Work out the finished part from the listing and answer in its coordinate system (mm). Coordinates: 2 decimals unless noted, no trailing zeros. Loops run counter-clockwise (first coordinate to the right, second up) from the corner with the lowest first, then second, coordinate; pieces in that order, holes last. Notation, with made-up numbers: (18.5, 61) -> (75.5, 61) arc R30 ccw to (75.5, 92) -> close; hole circle Ø8 at (28.5, -27.5). An arc over 180 degrees is marked (long way). Use a Markdown table: item, result. Add a question column.
```python
from build123d import *

# Parameters (mm, degrees)
F0_W         = 90
F0_H         = 60
F1_DEPTH     = 3
F2_R         = 2.5
F3_DEPTH     = 2
F4_R         = 1.5
F5_DEPTH     = 5
F6_R         = 7
F7_DEPTH     = 2.5
F8_R         = 5.25
F8_R_2       = 2.1
F9_DEPTH     = 4.3
F10_DEPTH    = 5.5
F11_W        = 31.5768257218
F11_H        = 6.5
F12_DEPTH    = 3
F13_T1_DEPTH = 3
F14_SIZE     = 1.5
F15_R        = 5
F16_R        = 3


# Not quite as in the source:
# - a fillet or chamfer that OpenCascade refuses, or shapes differently, is made with other operations: its cross-section is extruded or revolved along the edge and cut away or added


with BuildPart() as f1:
    # F0 (on Top) → F1 (new body)
    with BuildSketch(Plane.XY):
        Rectangle(F0_W, F0_H)
    extrude(amount=F1_DEPTH)

    # F2 (on face) → F3 (join)
    with BuildSketch(Plane.XY.offset(3)):
        with Locations((-39, 24.5)):
            Circle(F2_R)
        with Locations((19, 24.5)):
            Circle(F2_R)
        with Locations((19, -24.5)):
            Circle(F2_R)
        with Locations((-39, -24.5)):
            Circle(F2_R)
    extrude(amount=F3_DEPTH)

    # F4 (on face) → F5 (cut, through all)
    with BuildSketch(Plane(origin=(0, 0, 0), x_dir=(1, 0, 0), z_dir=(0, 0, -1))):
        with Locations((-39, 24.5)):
            Circle(F4_R)
        with Locations((19, 24.5)):
            Circle(F4_R)
        with Locations((19, -24.5)):
            Circle(F4_R)
        with Locations((-39, -24.5)):
            Circle(F4_R)
    extrude(amount=-F5_DEPTH, mode=Mode.SUBTRACT)

    # F6 (on face) → F7 (join)
    with BuildSketch(Plane(origin=(0, 0, 0), x_dir=(1, 0, 0), z_dir=(0, 0, -1))):
        with Locations((30, -17.5)):
            Circle(F6_R)
        with Locations((30, 17.5)):
            Circle(F6_R)
        with Locations((-30, -17.5)):
            Circle(F6_R)
        with Locations((-30, 17.5)):
            Circle(F6_R)
    extrude(amount=F7_DEPTH)

    # F8 (on face) → F9 (cut)
    with BuildSketch(Plane.XY.offset(3)):
        with Locations((30, -17.5)):
            Circle(F8_R)
        with Locations((30, -17.5)):
            Circle(F8_R_2, mode=Mode.SUBTRACT)
        with Locations((-30, -17.5)):
            Circle(F8_R)
        with Locations((-30, -17.5)):
            Circle(F8_R_2, mode=Mode.SUBTRACT)
        with Locations((-30, 17.5)):
            Circle(F8_R)
        with Locations((-30, 17.5)):
            Circle(F8_R_2, mode=Mode.SUBTRACT)
        with Locations((30, 17.5)):
            Circle(F8_R)
        with Locations((30, 17.5)):
            Circle(F8_R_2, mode=Mode.SUBTRACT)
    extrude(amount=-F9_DEPTH, mode=Mode.SUBTRACT)

    # F8 (on face) → F10 (cut, through all)
    with BuildSketch(Plane.XY.offset(3)):
        with Locations((-30, -17.5)):
            Circle(F8_R_2)
        with Locations((-30, 17.5)):
            Circle(F8_R_2)
        with Locations((30, 17.5)):
            Circle(F8_R_2)
        with Locations((30, -17.5)):
            Circle(F8_R_2)
    extrude(amount=-F10_DEPTH, mode=Mode.SUBTRACT)

    # F11 (on face) → F12 (cut, through all)
    with BuildSketch(Plane.XY.offset(3)):
        Polygon((-40, 17.5448150044), (-45, 20.4614816711), (-45, -20.4614816711), (-40, -17.5448150044), align=None)
        Polygon((-9.9231742782, 0), (-30, 11.7114816711), (-30, -11.7114816711), align=None)
        Polygon((20.0768257218, 17.5), (-20.0768257218, 17.5), (0, 5.7885183289), align=None)
        Polygon((0, -5.7885183289), (-20.0768257218, -17.5), (20.0768257218, -17.5), align=None)
        Polygon((30, 11.7114816711), (9.9231742782, 0), (30, -11.7114816711), align=None)
        Polygon((45, -20.4614816711), (45, 20.4614816711), (40, 17.5448150044), (40, -17.5448150044), align=None)
        with Locations((-4.2884128609, 26.75)):
            Rectangle(F11_W, F11_H)
        with Locations((-4.2884128609, -26.75)):
            Rectangle(F11_W, F11_H)
    extrude(amount=-F12_DEPTH, mode=Mode.SUBTRACT)

    # F13: fillet of radius 2 on 12 edges, made by hand

    # F13_s2 → F13_t1 (join)
    with BuildSketch(Plane.XY):
        with BuildLine():
            ThreePointArc((-26.992257949, -9.9569654746), (-28.9961214529, -9.963691978), (-30, -8.2294076728))
            Line((-30, -8.2294076728), (-30, -11.7114816711))
            Line((-30, -11.7114816711), (-26.992257949, -9.9569654746))
        make_face()
        with BuildLine():
            ThreePointArc((-26.992257949, 9.9569654746), (-28.9961214529, 9.963691978), (-30, 8.2294076728))
            Line((-30, 8.2294076728), (-30, 11.7114816711))
            Line((-30, 11.7114816711), (-26.992257949, 9.9569654746))
        make_face()
        with BuildLine():
            ThreePointArc((-12.8847019384, -1.7275578018), (-11.8924439894, 0), (-12.8847019384, 1.7275578018))
            Line((-12.8847019384, 1.7275578018), (-9.9231742782, 0))
            Line((-9.9231742782, 0), (-12.8847019384, -1.7275578018))
        make_face()
        with BuildLine():
            ThreePointArc((12.8847019384, 1.7275578018), (11.8924439894, 0), (12.8847019384, -1.7275578018))
            Line((12.8847019384, -1.7275578018), (9.9231742782, 0))
            Line((9.9231742782, 0), (12.8847019384, 1.7275578018))
        make_face()
        with BuildLine():
            ThreePointArc((30, -8.2294076728), (28.9961214529, -9.963691978), (26.992257949, -9.9569654746))
            Line((26.992257949, -9.9569654746), (30, -11.7114816711))
            Line((30, -11.7114816711), (30, -8.2294076728))
        make_face()
        with BuildLine():
            ThreePointArc((30, 8.2294076728), (28.9961214529, 9.963691978), (26.992257949, 9.9569654746))
            Line((26.992257949, 9.9569654746), (30, 11.7114816711))
            Line((30, 11.7114816711), (30, 8.2294076728))
        make_face()
        with BuildLine():
            ThreePointArc((12.678984582, 17.5), (14.6096730089, 16.0219599584), (13.686726633, 13.7724421982))
            Line((13.686726633, 13.7724421982), (20.0768257218, 17.5))
            Line((20.0768257218, 17.5), (12.678984582, 17.5))
        make_face()
        with BuildLine():
            ThreePointArc((12.678984582, -17.5), (14.6096730089, -16.0219599584), (13.686726633, -13.7724421982))
            Line((13.686726633, -13.7724421982), (20.0768257218, -17.5))
            Line((20.0768257218, -17.5), (12.678984582, -17.5))
        make_face()
        with BuildLine():
            ThreePointArc((-13.686726633, -13.7724421982), (-14.6096730089, -16.0219599584), (-12.678984582, -17.5))
            Line((-12.678984582, -17.5), (-20.0768257218, -17.5))
            Line((-20.0768257218, -17.5), (-13.686726633, -13.7724421982))
        make_face()
        with BuildLine():
            ThreePointArc((-12.678984582, 17.5), (-14.6096730089, 16.0219599584), (-13.686726633, 13.7724421982))
            Line((-13.686726633, 13.7724421982), (-20.0768257218, 17.5))
            Line((-20.0768257218, 17.5), (-12.678984582, 17.5))
        make_face()
        with BuildLine():
            ThreePointArc((-1.007742051, 6.3763678587), (0, 6.1039256605), (1.007742051, 6.3763678587))
            Line((1.007742051, 6.3763678587), (0, 5.7885183289))
            Line((0, 5.7885183289), (-1.007742051, 6.3763678587))
        make_face()
        with BuildLine():
            ThreePointArc((-1.007742051, -6.3763678587), (0, -6.1039256605), (1.007742051, -6.3763678587))
            Line((1.007742051, -6.3763678587), (0, -5.7885183289))
            Line((0, -5.7885183289), (-1.007742051, -6.3763678587))
        make_face()
    extrude(amount=F13_T1_DEPTH)

    # F14
    f14_edges = [f1.edges().sort_by_distance(p)[0] for p in [
        (11.5, -23.5, 1.5),
        (-20.076826, -23.5, 1.5),
        (11.5, 23.5, 1.5),
        (-20.076826, 23.5, 1.5),
    ]]
    chamfer(f14_edges, length=F14_SIZE)

    # F15
    f15_edges = [f1.edges().sort_by_distance(p)[0] for p in [
        (45, -30, 1.5),
        (45, 30, 1.5),
        (-45, 30, 1.5),
        (-45, -30, 1.5),
    ]]
    fillet(f15_edges, radius=F15_R)

    # F16
    f16_edges = [f1.edges().sort_by_distance(p)[0] for p in [
        (11.5, -30, 1.5),
        (-20.076826, 30, 1.5),
        (11.5, 30, 1.5),
        (-20.076826, -30, 1.5),
    ]]
    fillet(f16_edges, radius=F16_R)


solid = f1.part
```
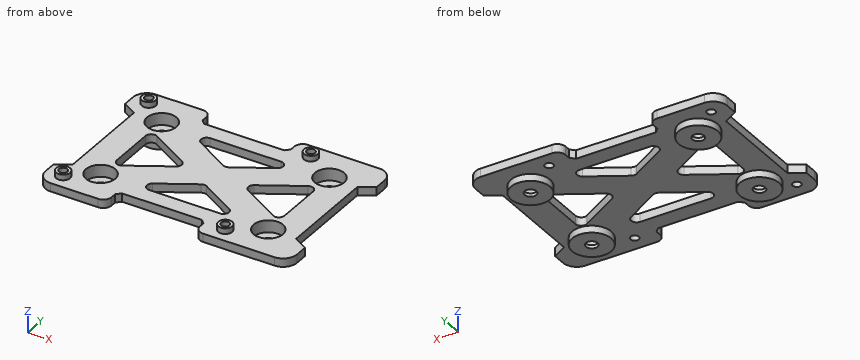
Item 1: Section A-A (x = -39) is taken. Determine the outline of the cut face in (y, z).
Item 2: Section C-C (x = 19) is taken. Determine the outline of the cut face in (y, z).
Item 3: Find the intervals of material crossed by probe 1 along Y at (x, z) = (-39, 1.4); probe 2 along Y at (x, z) = (-30, -2.25); probe 3 along Y at (x, z) = (20, 3.25), in increasing order.
Item 4: Section B-B (y = 3) is taken. Determine the outline of the cut face in (x, z).
Item 5: Section D-D (z = 1) is taken. Count the separate pieces of the cut face and the enclosed holes in it, then the cut area to 3 significant figures.
Item 6: Given pin 1 (1.5 mm diameter, centred on x = -7.5, z = 1.5, fed in from +Y); pin 2 (12 mm diameter, centred on x = -30, y = -17.5, fed in from +Z); pin 3 (0.9 mm diameter, centred on x = -9.5, z = 1.5, fed in from -Y); pin 4 (4 mm diameter, centred on x = 30, y = -17.5, fed in from +Z), each flat-ended and moving along its own axis, determine where each tip first touches the part or whether it passes through.
Output:
| question | item | result |
|---|---|---|
| 1 | outline | (-30, 0) -> (-26, 0) -> (-26, 5) -> (-27, 5) -> (-27, 3) -> (-30, 3) -> close; (-23, 0) -> (23, 0) -> (23, 5) -> (22, 5) -> (22, 3) -> (-22, 3) -> (-22, 5) -> (-23, 5) -> close; (26, 0) -> (30, 0) -> (30, 3) -> (27, 3) -> (27, 5) -> (26, 5) -> close |
| 2 | outline | (-30, 0) -> (-26, 0) -> (-26, 5) -> (-27, 5) -> (-27, 3) -> (-30, 3) -> close; (-23, 0) -> (-5.29, 0) -> (-5.29, 3) -> (-22, 3) -> (-22, 5) -> (-23, 5) -> close; (5.29, 0) -> (23, 0) -> (23, 5) -> (22, 5) -> (22, 3) -> (5.29, 3) -> close; (26, 0) -> (30, 0) -> (30, 3) -> (27, 3) -> (27, 5) -> (26, 5) -> close |
| 3 | probe 1 | y = -30 to -26, -23 to 23, 26 to 30 |
| 3 | probe 2 | y = -24.5 to -19.6, -15.4 to -10.5, 10.5 to 15.4, 19.6 to 24.5 |
| 3 | probe 3 | y = -26.79 to -25.62, -23.38 to -22.21, 22.21 to 23.38, 25.62 to 26.79 |
| 4 | outline | (-40, 0) -> (-30, 0) -> (-30, 3) -> (-40, 3) -> close; (-15.07, 0) -> (15.07, 0) -> (15.07, 3) -> (-15.07, 3) -> close; (30, 0) -> (40, 0) -> (40, 3) -> (30, 3) -> close |
| 5 | separate pieces | 1 |
| 5 | enclosed holes | 12 |
| 5 | area | 3,320 mm2 |
| 6 | pin 1 | stops at y = 23.5 |
| 6 | pin 2 | stops at z = 3 |
| 6 | pin 3 | stops at y = -23.5 |
| 6 | pin 4 | passes through |
